Design review of the part built by this model. Coordinates are the model's own, in mm. Give positions to 0.01 mm unless a question says otherwise; leave off trailing zeros. Order: outer loops, then holes, each group sorted by start corner. A loop starts at its lowest first (then second) coordinate and runs counter-clockwise, first axis right, second up. Notation, with made-up numbers: M 63,-29.5 L 113,-29.5 A25 ccw 113,5.5 Z; hole C -6,37.5 d5. An arc over 180 degrees is marked long. Answer as a JSON object with one key per item and string values.
from build123d import *

# Parameters (mm, degrees)
SZKIC1_R                    = 3.9
DODANIE_WYCI_GNI_CIE1_DEPTH = 114
SZKIC4_W                    = 2
SZKIC4_H                    = 5
OBR_T1_ANGLE                = 30
ZAOKR_GLENIE5_R             = 0.5
WYTNIJ_WYCI_GNI_CIE1_DEPTH  = 114
WYTNIJ_WYCI_GNI_CIE2_DEPTH  = 11.5


with BuildPart() as part:
    # Szkic1 → Dodanie-wyci_gni_cie1 (new body)
    with BuildSketch(Plane.XY):
        Circle(SZKIC1_R)
    extrude(amount=DODANIE_WYCI_GNI_CIE1_DEPTH)

    # Szkic4 → Obr_t1 (revolve)
    with BuildSketch(Plane(origin=(0, 0, 0), x_dir=(0, 0, -1), z_dir=(1, 0, 0))):
        with Locations((-74.25, 2.217381868)):
            Rectangle(SZKIC4_W, SZKIC4_H)
        with Locations((-35.75, 2.217381868)):
            Rectangle(SZKIC4_W, SZKIC4_H)
    revolve(axis=Axis((0, -0.282618132, 75.25), (0, 0, -1)), revolution_arc=OBR_T1_ANGLE)

    # Zaokr_glenie5
    zaokr_glenie5_edges = [part.edges().sort_by_distance(p)[0] for p in [
        (2.5, 4.047508887, 35.75),
        (0, 4.308690934, 36.75),
        (2.285548402, 3.676067824, 36.75),
        (1.294095226, 4.547010999, 36.75),
        (0, 4.717381868, 35.75),
        (2.285548402, 3.676067824, 73.25),
        (0, 4.717381868, 74.25),
        (0, 4.308690934, 73.25),
        (2.5, 4.047508887, 74.25),
        (1.294095226, 4.547010999, 73.25),
    ]]
    fillet(zaokr_glenie5_edges, radius=ZAOKR_GLENIE5_R)

    # Szkic5 → Wytnij-wyci_gni_cie1 (cut)
    with BuildSketch(Plane.XY.offset(114)):
        with BuildLine():
            Line((2.24849307, -0.185145655), (1.947595825, -1.138802222))
            ThreePointArc((1.947595825, -1.138802222), (1.994182967, -1.672529674), (2.404527351, -2.016989891))
            Line((2.404527351, -2.016989891), (3.548915231, -2.378066585))
            Line((3.548915231, -2.378066585), (3.909991925, -1.233678704))
            Line((3.909991925, -1.233678704), (4.271068619, -0.089290824))
            Line((4.271068619, -0.089290824), (3.126680739, 0.27178587))
            ThreePointArc((3.126680739, 0.27178587), (2.592953287, 0.225198729), (2.24849307, -0.185145655))
        make_face()
    extrude(amount=-WYTNIJ_WYCI_GNI_CIE1_DEPTH, mode=Mode.SUBTRACT)

    # Szkic5_3 → Wytnij-wyci_gni_cie2 (cut)
    with BuildSketch(Plane.XY.offset(114)):
        with BuildLine():
            Line((-3.66646605, 2.192493262), (-2.505030255, 1.890720345))
            ThreePointArc((-2.505030255, 1.890720345), (-2.077521655, 1.567808977), (-2.003560242, 1.03718193))
            Line((-2.003560242, 1.03718193), (-2.255037673, 0.069318767))
            ThreePointArc((-2.255037673, 0.069318767), (-2.577949041, -0.358189833), (-3.108576089, -0.432151245))
            Line((-3.108576089, -0.432151245), (-4.270011884, -0.130378328))
            Line((-4.270011884, -0.130378328), (-3.968238967, 1.031057467))
            Line((-3.968238967, 1.031057467), (-3.66646605, 2.192493262))
        make_face()
    extrude(amount=-WYTNIJ_WYCI_GNI_CIE2_DEPTH, mode=Mode.SUBTRACT)


solid = part.part
(1) Insertion check: pin 1 (0.6 mm diameter, centred on x = -3, y = 1, fed in from +Z); pin 2 (1.5 mm diameter, centred on y = -1.5, z = 85, fed in from -X). Each pin has a flat end and moves straight along its axis. Give the tip position at first contact, or say it passes through.
Checked values:
{"pin 1": "stops at z = 102.5", "pin 2": "stops at x = -3.83"}
(2) We need section A-A (z = 16.5). Write out the cut boundary in (x, y).
Checked values:
{"outline": "M 1.95,-1.14 L 2.25,-0.19 A0.7 cw 3.13,0.27 L 3.9,0.03 A3.9 ccw long 3.18,-2.26 L 2.4,-2.02 A0.7 cw Z"}
(3) To check wall thickness, follow L1, parallel to X at y = -0.25, z = 6.5; L2, parallel to X at y = 4.25, z = 36; L3, parallel to Z at x = -3.25, y = 1.5. State the ranges of each line that lie inside material, in increasing order. Write a range as from..to.
Checked values:
{"L1": "x = -3.89..2.23", "L2": "x = 0..2.09", "L3": "z = 0..102.5"}
